Design review of the part built by this model. Coordinates are the model's own, in mm. A direction names the side the tool comes from. Coordinates: 2 decimals unless noted, no trailing zeros. Loops run counter-clockwise (first coordinate to the right, second up) from the corner with the lowest first, then second, coordinate; pieces in that order, holes last.
from build123d import *

# Parameters (mm, degrees)
F0_W     = 508
F0_H     = 63.5
F1_DEPTH = 19.05
F3_DEPTH = 50.8
F5_DEPTH = 50.8
F7_DEPTH = 38.1
F9_DEPTH = 38.1


with BuildPart() as f1:
    # F0 (on Front) → F1 (new body)
    with BuildSketch(Plane.XZ):
        with Locations((7.0352284261, 31.75)):
            Rectangle(F0_W, F0_H)
    extrude(amount=F1_DEPTH)

    # F2 (on face) → F3 (cut)
    with BuildSketch(Plane.XZ.offset(19.05)):
        Polygon((-224.2599035735, 0), (-246.9647715739, 63.5), (-246.9647715739, 0), align=None)
    extrude(amount=-F3_DEPTH, mode=Mode.SUBTRACT)

    # F4 (on face) → F5 (cut)
    with BuildSketch(Plane.XZ.offset(19.05)):
        Polygon((261.0352284261, 0), (-237.0874956021, 35.8756586385), (-224.2599035735, 0), align=None)
    extrude(amount=-F5_DEPTH, mode=Mode.SUBTRACT)

    # F6 (on face) → F7 (cut)
    with BuildSketch(Plane.XZ.offset(19.05)):
        Polygon((238.3303604257, 63.5), (261.0352284261, 0), (261.0352284261, 63.5), align=None)
    extrude(amount=-F7_DEPTH, mode=Mode.SUBTRACT)

    # F8 (on face) → F9 (cut)
    with BuildSketch(Plane(origin=(231.445604258, 0, 82.7549904558), x_dir=(0, 1, 0), z_dir=(0.941618337, 0, 0.3366822055))):
        Polygon((-19.05, 40.5242251848), (-19.05, -87.885916413), (-9.525, -87.885916413), (-9.525, 37.3283624649), align=None)
    extrude(amount=-F9_DEPTH, mode=Mode.SUBTRACT)


solid = f1.part
Q1. Machinability: for faces 1 (the flat face through (15.461, -9.658, 17.687)), 2 (the flat face through (208.534, -14.354, 33.669)), which of the approach directions +Z, -Z, +X, -X, +Y, -Y give a long, thin tool a straight path to every point of the face, cutting with its end or side? Answer none if there is none.
Q2. Take a section at D-D, the plane z = 55. Write out the cut boundary in (x, y) (3 decimals).
Q3. Take a section at B-B, the plane z = 10.5. Write out the cut boundary in (x, y) (3 decimals), then the cut area to 3 significant figures.
Q4. For line 1 (Z direction, x = 189.5, y = -13.25); line 2 (X direction, y = -2.75, z = 55); line 3 (Z direction, x = -138.5, y = -8), list the stretches that pass through material, from the lowest coordinate up.
Q5. Take a section at C-C, the plane x = 93. Write out the cut boundary in (y, z), then the cut area to 3 significant figures.
Q6. Take a section at A-A, the plane y = -13.25. Write out the cut boundary in (x, z), then the cut area to 3 significant figures.
Q7. Clearance check with flat-ended pins moving along their axes: pin 1 Ø8 at (x, y) = (120.5, -15) entering from -Z; pin 2 Ø5 at (y, z) = (-9.5, 35) entering from +X; pin 3 Ø1.5 at (x, y) = (12, -8) entering from -Z. State where each tip first meets the part, or that it passes through.
Entries:
1. face 1: -Z, -X, +Y, -Y
1. face 2: +Z, +X, -Y
2. outline: (-243.926, -19.05) - (200.907, -19.05) - (200.907, -9.525) - (241.37, -9.525) - (241.37, 0) - (-243.926, 0) - close
3. outline: (115.246, -19.05) - (216.819, -19.05) - (216.819, -9.525) - (257.281, -9.525) - (257.281, 0) - (115.246, 0) - close
3. area: 2,320 mm2
4. line 1: z = 5.15 to 63.5
4. line 2: x = -243.93 to 241.37
4. line 3: z = 28.78 to 63.5
5. outline: (-19.05, 12.1) - (0, 12.1) - (0, 63.5) - (-19.05, 63.5) - close
5. area: 979 mm2
6. outline: (-246.96, 63.5) - (-237.09, 35.88) - (219.5, 2.99) - (197.87, 63.5) - close
6. area: 19,600 mm2
7. pin 1: stops at z = 9.83
7. pin 2: stops at x = 249.41
7. pin 3: stops at z = 17.88
